from build123d import *

# Parameters (mm, degrees)
F0_W     = 63.5
F0_H     = 63.5
F1_DEPTH = 6.35
F2_R     = 5.08
F4_D     = 5.08
F5_R     = 2.54
F6_DEPTH = 25.4
F7_W     = 46.99
F7_H     = 46.99
F7_W_2   = 38.1
F7_H_2   = 38.1
F8_DEPTH = 25.4
F9_R     = 5.08
F10_R    = 3.81


with BuildPart() as f1:
    # F0 (on Top) → F1 (new body)
    with BuildSketch(Plane.XY):
        Rectangle(F0_W, F0_H)
    extrude(amount=F1_DEPTH)

    # F2
    f2_edges = [f1.edges().sort_by_distance(p)[0] for p in [
        (-31.75, -31.75, 3.175),
        (31.75, -31.75, 3.175),
        (31.75, 31.75, 3.175),
        (-31.75, 31.75, 3.175),
    ]]
    fillet(f2_edges, radius=F2_R)

    # F4 (through all)
    with Locations(Plane.XY.offset(6.35)):
        with Locations((-26.67, 26.67), (26.67, 26.67), (26.67, -26.67), (-26.67, -26.67)):
            Hole(F4_D / 2)

    # F5 (on face) → F6 (join)
    with BuildSketch(Plane(origin=(0, 31.75, 0), x_dir=(-1, 0, 0), z_dir=(0, 1, 0))):
        with Locations((0, 3.175)):
            Circle(F5_R)
    extrude(amount=F6_DEPTH)

    # F7 (on face) → F8 (join)
    with BuildSketch(Plane.XY.offset(6.35)):
        Rectangle(F7_W, F7_H)
        Rectangle(F7_W_2, F7_H_2, mode=Mode.SUBTRACT)
    extrude(amount=F8_DEPTH)

    # F9
    f9_edges = [f1.edges().sort_by_distance(p)[0] for p in [
        (-23.495, -23.495, 19.05),
        (23.495, -23.495, 19.05),
        (23.495, 23.495, 19.05),
        (-23.495, 23.495, 19.05),
    ]]
    fillet(f9_edges, radius=F9_R)

    # F10
    f10_edges = [f1.edges().sort_by_distance(p)[0] for p in [
        (19.05, 19.05, 19.05),
        (-19.05, 19.05, 19.05),
        (-19.05, -19.05, 19.05),
        (19.05, -19.05, 19.05),
    ]]
    fillet(f10_edges, radius=F10_R)


solid = f1.part
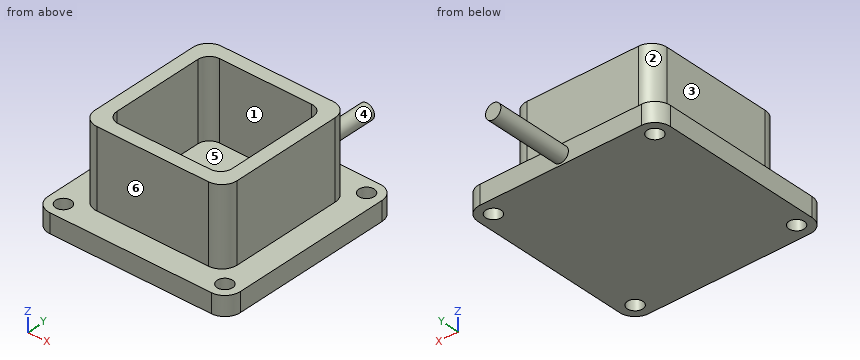
The listing builds one solid part. Answer for the finished solid, in the listing's coordinates (mm). Face numbers are marked on the shaded views. A direction names the side the tool comes from. Give positions to 0.01 mm unless a question says otherwise; leave off trailing zeros. Order: outer loops, then holes, each group sorted by start corner. A loop starts at its lowest first (then second) coordinate and runs counter-clockwise, first axis right, second up. Notation, with made-up numbers: (53.25, -7.75) - (64.25, -7.75) arc R23 ccw to (64.25, 13.25) - close; hole circle Ø6 at (-27.75, 2.5). An arc over 180 degrees is marked (long way). Answer as CSV lines item,"result".
Q1. Each of these flat-tipped pins is pushed along its axis until it touches: pin 1 Ø8 at (x, y) = (-8, 0) entering from +Z; pin 2 Ø7.5 at (x, z) = (2, 20) entering from -Y (3 decimals); pin 3 Ø12 at (x, z) = (9, 10.5) entering from +Y; pin 4 Ø8 at (x, y) = (15, -1) entering from -Z. Where does it stop, or does it pass through?
Answer key:
pin 1,"stops at z = 6.35"
pin 2,"stops at y = -23.495"
pin 3,"stops at y = 31.75"
pin 4,"stops at z = 0"
Q2. A cutting plane is placed at D-D, the plane x = 21. Determine the outline of the cut face in (y, z).
Answer key:
outline,"(-31.75, 0) - (31.75, 0) - (31.75, 6.35) - (22.79, 6.35) - (22.79, 31.75) - (-22.79, 31.75) - (-22.79, 6.35) - (-31.75, 6.35) - close"
Q3. A cutting plane is placed at B-B, the plane z = 29. Determine the outline of the cut face in (x, y) (3 decimals).
Answer key:
outline,"(-23.495, -18.415) arc R5.08 ccw to (-18.415, -23.495) - (18.415, -23.495) arc R5.08 ccw to (23.495, -18.415) - (23.495, 18.415) arc R5.08 ccw to (18.415, 23.495) - (-18.415, 23.495) arc R5.08 ccw to (-23.495, 18.415) - close; hole (-19.05, -15.24) arc R3.81 ccw to (-15.24, -19.05) - (15.24, -19.05) arc R3.81 ccw to (19.05, -15.24) - (19.05, 15.24) arc R3.81 ccw to (15.24, 19.05) - (-15.24, 19.05) arc R3.81 ccw to (-19.05, 15.24) - close"
Q4. Which of the six approach directions +Z, -Z, +X, -X, +Y, -Y give full straight-line access (tool end or side, diameter ignored) to the marked faces 4, 5 and 6?
Answer key:
face 4,"+Y"
face 5,"+Z"
face 6,"+Z, +X, -X, -Y"
Q5. Determine the mould class of the marked faces 1, 2 and 3 for opening direction Y: pulls with the +Y half, pulls with the -Y half, needs draft (parallel to the pull), parting line crosses it, or undercut.
Answer key:
face 1,"undercut"
face 2,"pulls with the +Y half"
face 3,"needs draft"
Q6. Straight lines are drawn through the part: L1, parallel to Y at x = 26.67, z = 4; L2, parallel to Y at x = -11, z = 17 (3 decimals). For each, find the intervals that lie inside material, in ascending order.
Answer key:
L1,"y = -31.75 to -29.21, -24.13 to 24.13, 29.21 to 31.75"
L2,"y = -23.495 to -19.05, 19.05 to 23.495"
Q7. A cutting plane is placed at A-A, the plane x = 6. Determine the outline of the cut face in (y, z) (3 decimals).
Answer key:
outline,"(-31.75, 0) - (31.75, 0) - (31.75, 6.35) - (23.495, 6.35) - (23.495, 31.75) - (19.05, 31.75) - (19.05, 6.35) - (-19.05, 6.35) - (-19.05, 31.75) - (-23.495, 31.75) - (-23.495, 6.35) - (-31.75, 6.35) - close"
Q8. A cutting plane is placed at C-C, the plane y = -16.5. Determine the outline of the cut face in (x, z) (3 decimals), and give its area (3 significant figures).
Answer key:
outline,"(-31.75, 0) - (31.75, 0) - (31.75, 6.35) - (23.495, 6.35) - (23.495, 31.75) - (18.836, 31.75) - (18.836, 6.35) - (-18.836, 6.35) - (-18.836, 31.75) - (-23.495, 31.75) - (-23.495, 6.35) - (-31.75, 6.35) - close"
area,"640 mm^2"
